Verification items for the finished model (mm, model axes). A direction names the side the tool comes from. Coordinates: 2 decimals unless noted, no trailing zeros. Order: outer loops, then holes, each group sorted by start corner. A loop starts at its lowest first (then second) coordinate and runs counter-clockwise, first axis right, second up. Notation, with made-up numbers: M 81.5,-2.75 L 99.5,-2.75 A22 cw 99.5,7.25 Z; hole C 69,-21 d10. An arc over 180 degrees is marked long. Return JSON: item names as keys, results as strings. Group by question number.
1. Section check B-B, the plane z = 22. Record the cut outline in (x, y), plus the area to 3 significant figures.
2. Section check D-D, the plane x = 52. Record the cut outline in (y, z).
3. Mould release check, pull along X, two halves, no side actions. Record for faces 1 (the flat face through (51.257, 10, 10)), 2 (the flat face through (10, 0, 18)), 3 (the flat face through (31, 20, 13)), 4 (the flat face through (51.257, 15, 28)): +X half, -X half, draft (parallel to the pull), parting line (faces both ways), or undercut.
4. Gauge pin test, flat ends, axial feed: pin 1 (1.5 mm diameter, centred on x = 23, z = 11, fed in from -Y); pin 2 (12 mm diameter, centred on y = 14, z = 5.5, fed in from +X); pin 3 (8 mm diameter, centred on x = 60.5, z = 7.5, fed in from +Y). Record the tip position at first contact, or that the pin passes through.
5. Section check A-A, the plane y = 19. Record the cut outline in (x, z).
6. Section check C-C, the plane y = 3.25. Record the cut outline in (x, z), plus the area to 3 significant figures.
7. Set-up check for faces 5 (the flat face through (59, 4, 10)), 6 (the flat face through (31, 10, 27.29)), 7 (the flat face through (4, 4, 10)), 8 (the flat face through (11.257, 10, 13)): record each of +Z, -Z, +X, -X, +Y, -Y from which the full face is reachable in a straight line by a thin tool's end or side.
8. Material ranges on line 1 along X through (y, z) = (11.5, 16); line 2 along Z through (x, y) = (54, 8); line 3 along Z through (x, y) = (36, 13.5), recorded low to high.
```python
from build123d import *

# Parameters (mm, degrees)
BOSS_EXTRUDE1_DEPTH = 20
BOSS_EXTRUDE2_DEPTH = 4
BOSS_EXTRUDE3_DEPTH = 44


with BuildPart() as part:
    # Sketch1 → Boss-Extrude1 (new body)
    with BuildSketch(Plane.XY):
        Polygon((0, 0), (11.25748503, 0), (11.25748503, 20), (51.25748503, 20), (51.25748503, 0), (62.51497006, 0), (62.51497006, 4), (55.25748503, 4), (55.25748503, 24), (7.25748503, 24), (7.25748503, 4), (0, 4), align=None)
    extrude(amount=BOSS_EXTRUDE1_DEPTH)

    # Sketch2 → Boss-Extrude2 (add)
    with BuildSketch(Plane.ZY.offset(-7.25748503)):
        Polygon((27.29, 20), (20, 20), (20, 4), (20, 0), (27.29, 0), align=None)
        Polygon((20, 24), (20, 20), (27.29, 20), (27.29, 0), (31.29, 0), (31.29, 24), align=None)
    extrude(amount=-BOSS_EXTRUDE2_DEPTH)

    # Sketch2<3> → Boss-Extrude3 (add)
    with BuildSketch(Plane.ZY.offset(-7.25748503)):
        Polygon((20, 24), (20, 20), (27.29, 20), (27.29, 0), (31.29, 0), (31.29, 24), align=None)
    extrude(amount=-BOSS_EXTRUDE3_DEPTH)


solid = part.part
```
Answers follow:
{
 "1": {"outline": "M 7.26,0 L 11.26,0 L 11.26,20 L 51.26,20 L 51.26,24 L 7.26,24 Z", "area": "256 mm^2"},
 "2": {"outline": "M 0,0 L 24,0 L 24,20 L 0,20 Z"},
 "3": {"face 1": "undercut", "face 2": "draft", "face 3": "undercut", "face 4": "+X half"},
 "4": {"pin 1": "y = 20", "pin 2": "x = 55.26", "pin 3": "y = 4"},
 "5": {"outline": "M 7.26,0 L 11.26,0 L 11.26,27.29 L 51.26,27.29 L 51.26,31.29 L 7.26,31.29 Z; M 51.26,0 L 55.26,0 L 55.26,20 L 51.26,20 Z"},
 "6": {"outline": "M 0,0 L 11.26,0 L 11.26,27.29 L 51.26,27.29 L 51.26,31.29 L 7.26,31.29 L 7.26,20 L 0,20 Z; M 51.26,0 L 62.51,0 L 62.51,20 L 51.26,20 Z", "area": "655 mm^2"},
 "7": {"face 5": "+Z, -Z, +X, +Y", "face 6": "-Z, +X, -Y", "face 7": "+Z, -Z, -X, +Y", "face 8": "-Z, -Y"},
 "8": {"line 1": "7.26 to 11.26, 51.26 to 55.26", "line 2": "0 to 20", "line 3": "27.29 to 31.29"}
}
